from build123d import *

# Parameters (mm, degrees)
SKETCH1_W           = 40.2
SKETCH1_H           = 100
BOSS_EXTRUDE1_DEPTH = 10
SKETCH7_W           = 40.2
SKETCH7_H           = 96.8
CUT_EXTRUDE5_DEPTH  = 2.5
SKETCH4_W           = 40.2
SKETCH4_H           = 57
CUT_EXTRUDE1_DEPTH  = 5.6
SKETCH3_W           = 29
SKETCH3_H           = 31.2
CUT_EXTRUDE2_DEPTH  = 11
SKETCH2_R           = 1.35
CUT_EXTRUDE3_DEPTH  = 11
CUT_EXTRUDE4_REACH  = 102
SKETCH6_R           = 1.35


with BuildPart() as part:
    # Sketch1 → Boss-Extrude1 (new body)
    with BuildSketch(Plane.XY):
        Rectangle(SKETCH1_W, SKETCH1_H)
    extrude(amount=BOSS_EXTRUDE1_DEPTH)

    # Sketch7 → Cut-Extrude5 (cut)
    with BuildSketch(Plane.XY.offset(10)):
        with Locations((0, -1.6)):
            Rectangle(SKETCH7_W, SKETCH7_H)
    extrude(amount=-CUT_EXTRUDE5_DEPTH, mode=Mode.SUBTRACT)

    # Sketch4 → Cut-Extrude1 (cut)
    with BuildSketch(Plane.XY.offset(10)):
        with Locations((0, 18.5)):
            Rectangle(SKETCH4_W, SKETCH4_H)
    extrude(amount=-CUT_EXTRUDE1_DEPTH, mode=Mode.SUBTRACT)

    # Sketch3 → Cut-Extrude2 (cut, through all)
    with BuildSketch(Plane.XY.offset(10)):
        with Locations((0, -34.4)):
            Rectangle(SKETCH3_W, SKETCH3_H)
    extrude(amount=-CUT_EXTRUDE2_DEPTH, mode=Mode.SUBTRACT)

    # Sketch2 → Cut-Extrude3 (cut, through all)
    with BuildSketch(Plane.XY.offset(10)):
        with Locations((17.3, -23.8)):
            Circle(SKETCH2_R)
        with Locations((11, -16)):
            Circle(SKETCH2_R)
        with Locations((-17.3, -23.8)):
            Circle(SKETCH2_R)
        with Locations((-11, -16)):
            Circle(SKETCH2_R)
        with Locations((-17.3, -45.8)):
            Circle(SKETCH2_R)
        with Locations((17.3, -45.8)):
            Circle(SKETCH2_R)
    extrude(amount=-CUT_EXTRUDE3_DEPTH, mode=Mode.SUBTRACT)

    # Sketch6 → Cut-Extrude4 (cut, up to next)
    with BuildSketch(Plane(origin=(0, 50, 0), x_dir=(-1, 0, 0), z_dir=(0, 1, 0)), mode=Mode.PRIVATE) as cut_extrude4_sk1:
        with Locations((-11, 7.2)):
            Circle(SKETCH6_R)
    cut_extrude4_tool1 = extrude(cut_extrude4_sk1.sketch, amount=-CUT_EXTRUDE4_REACH, mode=Mode.PRIVATE) & part.part
    add(cut_extrude4_tool1.solids().sort_by_distance((11, 50, 7.2))[0], mode=Mode.SUBTRACT)
    # Sketch6 → Cut-Extrude4 (cut, up to next)
    with BuildSketch(Plane(origin=(0, 50, 0), x_dir=(-1, 0, 0), z_dir=(0, 1, 0)), mode=Mode.PRIVATE) as cut_extrude4_sk2:
        with Locations((11, 7.2)):
            Circle(SKETCH6_R)
    cut_extrude4_tool2 = extrude(cut_extrude4_sk2.sketch, amount=-CUT_EXTRUDE4_REACH, mode=Mode.PRIVATE) & part.part
    add(cut_extrude4_tool2.solids().sort_by_distance((-11, 50, 7.2))[0], mode=Mode.SUBTRACT)


solid = part.part
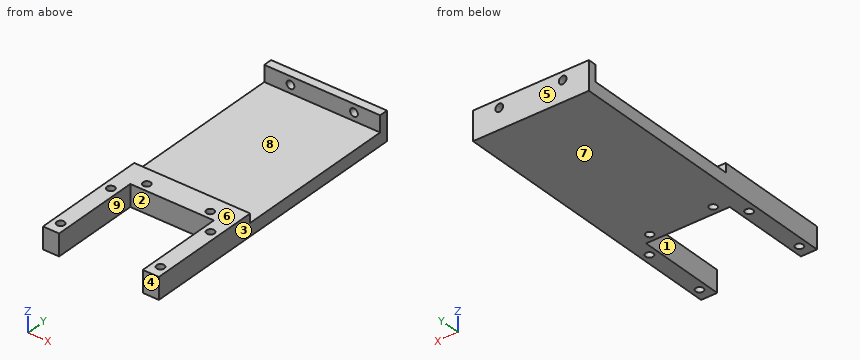
Check sheet for the modelled part. Datum: model origin and axes. Units: mm. Face numbers are marked on the shaded views. A direction names the side the tool comes from. Round coordinates to 2 decimals unless told otherwise and drop trailing zeros. Loops run counter-clockwise (first coordinate to the right, second up) from the corner with the lowest first, then second, coordinate; pieces in that order, holes last. Notation, with made-up numbers: (-29.75, 20.5) - (4.25, 20.5) arc R7 ccw to (4.25, 24.5) - close; hole circle Ø6 at (14.25, 39). An arc over 180 degrees is marked (long way). Answer as CSV lines item,"result". Start each with the question number.
Item 1: Section check D-D (x = 6.5). Record the boundary of the cut face in (y, z).
Item 2: Depth check by flat-ended pin: P1, Ø2, axis at x = -1, z = 3.5, coming from the -Y side; P2, Ø1, axis at x = -5, y = 28, coming from the +Z side; P3, Ø3, axis at x = -11, y = -16, coming from the +Z side. Enter the tip coordinate at first touch or a pass-through.
Item 3: Scan lines: line 1 (Y direction, x = 17.3, z = 2); line 2 (Y direction, x = -17.3, z = 5); line 3 (Y direction, x = -1.5, z = 6.75). Record each from-to range of solid material in increasing order. Write a range as [from, to].
Item 4: Set-up check for the marked faces 5, 6, 7, 8 and 9: record each of +Z, -Z, +X, -X, +Y, -Y from which the full face is reachable in a straight line by a thin tool's end or side.
Item 5: Section check B-B (x = 11). Record the boundary of the cut face in (y, z).
Item 6: Release check for a two-part mould opening along X. For the marked faces 1, 2, 3 and 4 record: +X half, -X half, draft (parallel to the pull), parting line (faces both ways), or undercut.
Item 7: Section check A-A (y = -23.8). Record the boundary of the cut face in (x, z).
Item 8: Section check C-C (z = 3.25). Record the boundary of the cut face in (x, y).
Report:
1,outline,"(-18.8, 0) - (50, 0) - (50, 10) - (47, 10) - (47, 4.4) - (-10, 4.4) - (-10, 7.5) - (-18.8, 7.5) - close"
2,P1,"stops at y = -18.8"
2,P2,"stops at z = 4.4"
2,P3,"stops at z = 7.5"
3,line 1,"y = [-50, -47.15], [-44.45, -25.15], [-22.45, 50]"
3,line 2,"y = [-50, -47.15], [-44.45, -25.15], [-22.45, -10], [47, 50]"
3,line 3,"y = [-18.8, -10], [47, 50]"
4,face 5,"+Z, -Z, +X, -X, +Y"
4,face 6,"+Z, +X, -X, -Y"
4,face 7,"-Z, +X, -X, +Y, -Y"
4,face 8,"+Z, +X, -X"
4,face 9,"+Z, -Z, -Y"
5,outline,"(-18.8, 0) - (-17.35, 0) - (-17.35, 7.5) - (-18.8, 7.5) - close; (-14.65, 0) - (50, 0) - (50, 5.85) - (47, 5.85) - (47, 4.4) - (-10, 4.4) - (-10, 7.5) - (-14.65, 7.5) - close; (47, 8.55) - (50, 8.55) - (50, 10) - (47, 10) - close"
6,face 1,"undercut"
6,face 2,"undercut"
6,face 3,"+X half"
6,face 4,"draft"
7,outline,"(-20.1, 0) - (-18.65, 0) - (-18.65, 7.5) - (-20.1, 7.5) - close; (-15.95, 0) - (-14.5, 0) - (-14.5, 7.5) - (-15.95, 7.5) - close; (14.5, 0) - (15.95, 0) - (15.95, 7.5) - (14.5, 7.5) - close; (18.65, 0) - (20.1, 0) - (20.1, 7.5) - (18.65, 7.5) - close"
8,outline,"(-20.1, -50) - (-14.5, -50) - (-14.5, -18.8) - (14.5, -18.8) - (14.5, -50) - (20.1, -50) - (20.1, 50) - (-20.1, 50) - close; hole circle Ø2.7 at (-17.3, -45.8); hole circle Ø2.7 at (-17.3, -23.8); hole circle Ø2.7 at (-11, -16); hole circle Ø2.7 at (11, -16); hole circle Ø2.7 at (17.3, -45.8); hole circle Ø2.7 at (17.3, -23.8)"
